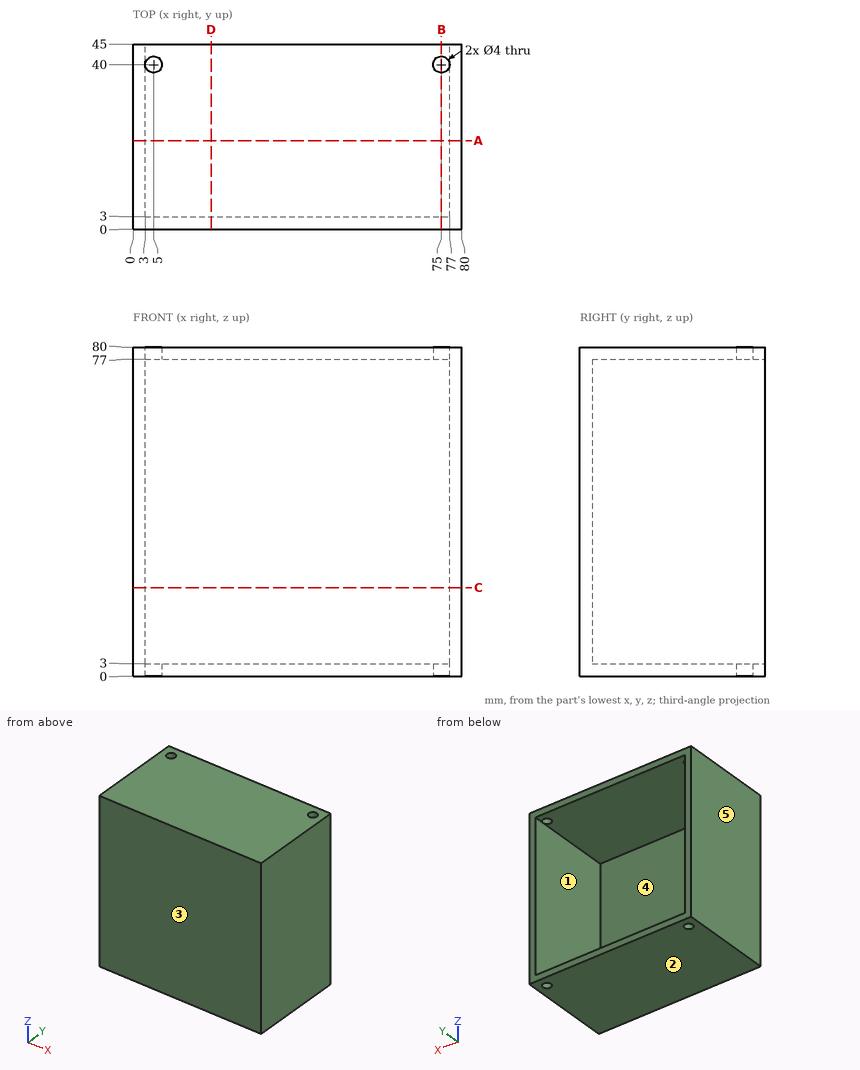
Design review of the part shown in the three views and the two pictorial views. Dimensions are in mm from the part's minimum x, y and z. A direction names the side the tool comes from. Round coordinates to 2 decimals unless told otherwise and drop trailing zeros. Order: outer loops, then holes, each group sorted by start corner. A loop starts at its lowest first (then second) coordinate and runs counter-clockwise, first axis right, second up.
(1) Wall thickness on L1, parallel to Z at x = 50, y = 31; L2, parallel to Y at x = 75, z = 77.8: over which ranges is each line inside the solid? List them lowest first.
Working result:
L1: z = 0 to 3, 77 to 80
L2: y = 0 to 38, 42 to 45
(2) Take a section at B-B, the plane x = 75. State the section outline as (y, z) points.
Working result:
outline: (0, 0) - (38, 0) - (38, 3) - (3, 3) - (3, 77) - (38, 77) - (38, 80) - (0, 80) - close; (42, 0) - (45, 0) - (45, 3) - (42, 3) - close; (42, 77) - (45, 77) - (45, 80) - (42, 80) - close
(3) Tool access review of the marked faces 4 and 5: name each direction out of +Z, -Z, +X, -X, +Y, -Y from which nothing blocks a thin tool from reaching the whole face with its end or side.
Working result:
face 4: +Y
face 5: +Z, -Z, -X, +Y, -Y
(4) Take a section at D-D, the plane x = 19. State the section outline as (y, z) points, plus the area to 3 significant figures.
Working result:
outline: (0, 0) - (45, 0) - (45, 3) - (3, 3) - (3, 77) - (45, 77) - (45, 80) - (0, 80) - close
area: 492 mm2
(5) For P1, Ø8, axis at x = 21.5, z = 45.5, coming from the +Y side, flat-tipped, find the tip position at first contact; note if it passes through.
Working result:
P1: stops at y = 3
(6) Take a section at C-C, the plane z = 21.5. State the section outline as (x, y) points.
Working result:
outline: (0, 0) - (80, 0) - (80, 45) - (77, 45) - (77, 3) - (3, 3) - (3, 45) - (0, 45) - close
(7) Mouldability with a two-part tool opening along Z and no side actions: class the marked faces 1, 2 and 3 as released by +Z, released by -Z, zero draft, split by the parting line, or undercut.
Working result:
face 1: undercut
face 2: released by -Z
face 3: zero draft
(8) Take a section at A-A, the plane y = 21.5. State the section outline as (x, z) points, plus the area to 3 significant figures.
Working result:
outline: (0, 0) - (80, 0) - (80, 80) - (0, 80) - close; hole (3, 3) - (77, 3) - (77, 77) - (3, 77) - close
area: 924 mm2
